Can you work these out from the model? Positions are in its coordinate system, mm. A direction names the side the tool comes from. Coordinates: 2 decimals unless noted, no trailing zeros. Write each loop counter-clockwise with the first axis right and the second up, starting at its lowest first coordinate (ties: lowest second). Pieces come first, ordered by that corner, then holes. Notation, with made-up numbers: M 6,39.5 L 16,39.5 A38 cw 16,78.5 Z; hole C 38.5,-3.75 d11. An arc over 180 degrees is marked long. Use one line per item in the form item = value. Start each with the question number.
```python
from build123d import *

# Parameters (mm, degrees)
SKETCH1_R                = 27.852115
SKETCH1_R_2              = 4
BOSS_EXTRUDE1_DEPTH      = 20
BOSS_EXTRUDE2_DEPTH      = 15
BOSS_EXTRUDE2_DEPTH_BACK = 15
SKETCH2_R                = 2.5
SKETCH4_R                = 1.7
CUT_EXTRUDE1_DEPTH       = 8


with BuildPart() as part:
    # Sketch1 → Boss-Extrude1 (new body)
    with BuildSketch(Plane.XY):
        Circle(SKETCH1_R)
        Circle(SKETCH1_R_2, mode=Mode.SUBTRACT)
    extrude(amount=BOSS_EXTRUDE1_DEPTH)

    # Sketch2 → Boss-Extrude2 (add, two sides: drawn at the far end of the back side and taken through both)
    with BuildSketch(Plane.XY.offset(10).offset(-BOSS_EXTRUDE2_DEPTH_BACK)):
        with Locations((-15, 15)):
            Circle(SKETCH2_R)
        with Locations((15, 15)):
            Circle(SKETCH2_R)
        with Locations((15, -15)):
            Circle(SKETCH2_R)
        with Locations((-15, -15)):
            Circle(SKETCH2_R)
    extrude(amount=BOSS_EXTRUDE2_DEPTH + BOSS_EXTRUDE2_DEPTH_BACK)

    # Sketch4 → Cut-Extrude1 (cut, symmetric)
    with BuildSketch(Plane.XY.offset(10)):
        with Locations((27.852115, 0)):
            Circle(SKETCH4_R)
        with Locations((27.42897879, -4.836469014)):
            Circle(SKETCH4_R)
        with Locations((26.172426939, -9.525984364)):
            Circle(SKETCH4_R)
        with Locations((24.120639139, -13.9260575)):
            Circle(SKETCH4_R)
        with Locations((21.335957925, -17.902994426)):
            Circle(SKETCH4_R)
        with Locations((17.902994426, -21.335957925)):
            Circle(SKETCH4_R)
        with Locations((13.9260575, -24.120639139)):
            Circle(SKETCH4_R)
        with Locations((9.525984364, -26.172426939)):
            Circle(SKETCH4_R)
        with Locations((4.836469014, -27.42897879)):
            Circle(SKETCH4_R)
        with Locations((0, -27.852115)):
            Circle(SKETCH4_R)
        with Locations((-4.836469014, -27.42897879)):
            Circle(SKETCH4_R)
        with Locations((-9.525984364, -26.172426939)):
            Circle(SKETCH4_R)
        with Locations((-13.9260575, -24.120639139)):
            Circle(SKETCH4_R)
        with Locations((-17.902994426, -21.335957925)):
            Circle(SKETCH4_R)
        with Locations((-21.335957925, -17.902994426)):
            Circle(SKETCH4_R)
        with Locations((-24.120639139, -13.9260575)):
            Circle(SKETCH4_R)
        with Locations((-26.172426939, -9.525984364)):
            Circle(SKETCH4_R)
        with Locations((-27.42897879, -4.836469014)):
            Circle(SKETCH4_R)
        with Locations((-27.852115, 0)):
            Circle(SKETCH4_R)
        with Locations((-27.42897879, 4.836469014)):
            Circle(SKETCH4_R)
        with Locations((-26.172426939, 9.525984364)):
            Circle(SKETCH4_R)
        with Locations((-24.120639139, 13.9260575)):
            Circle(SKETCH4_R)
        with Locations((-21.335957925, 17.902994426)):
            Circle(SKETCH4_R)
        with Locations((-17.902994426, 21.335957925)):
            Circle(SKETCH4_R)
        with Locations((-13.9260575, 24.120639139)):
            Circle(SKETCH4_R)
        with Locations((-9.525984364, 26.172426939)):
            Circle(SKETCH4_R)
        with Locations((-4.836469014, 27.42897879)):
            Circle(SKETCH4_R)
        with Locations((0, 27.852115)):
            Circle(SKETCH4_R)
        with Locations((4.836469014, 27.42897879)):
            Circle(SKETCH4_R)
        with Locations((9.525984364, 26.172426939)):
            Circle(SKETCH4_R)
        with Locations((13.9260575, 24.120639139)):
            Circle(SKETCH4_R)
        with Locations((17.902994426, 21.335957925)):
            Circle(SKETCH4_R)
        with Locations((21.335957925, 17.902994426)):
            Circle(SKETCH4_R)
        with Locations((24.120639139, 13.9260575)):
            Circle(SKETCH4_R)
        with Locations((26.172426939, 9.525984364)):
            Circle(SKETCH4_R)
        with Locations((27.42897879, 4.836469014)):
            Circle(SKETCH4_R)
    extrude(amount=CUT_EXTRUDE1_DEPTH, both=True, mode=Mode.SUBTRACT)


solid = part.part
```
1) Please list where these lines run through material, in increasing order: line 1 (X direction, y = -20, z = 16.5); line 2 (Y direction, x = 0, z = 10.75); line 3 (Z direction, x = -2, y = -5).
2) Suppose I cut it at A-A on x = 0. Please give me the cut outline in (y, z), and give its area (3 significant figures).
3) If we mould it in two halves opening along X, with no side actions, what happens to faces 3 (the face through (9, 25, 2)), 4 (the face through (-15, -15, -5)), 5 (the face through (-8.979, 24.563, 9.888))? For each: +X half, -X half, draft (parallel to the pull), parting line (faces both ways), or undercut.
4) Suppose I cut it at B-B on z = -1.25. Please give me the cut outline in (x, y), and give its area (3 significant figures).
5) Which directions (+Z, -Z, +X, -X, +Y, -Y) give clear straight access to the entire face, cutting with the end or side of a thin tool? Please do faces 1 (the face through (-15, -15, 25)), 2 (the face through (22.67, -13.04, 9.89)).
6) Will these pins go through, and if not, where does the flat tip stop? pin 1 Ø0.8 at (x, y) = (-13.5, -24) entering from +Z; pin 2 Ø6 at (x, z) = (-5.5, 17) entering from +Y; pin 3 Ø3 at (x, y) = (20.5, -17.5) entering from -Z.
Computed values:
q1.line_1 = -19.38 to -18.95, -16.85 to 16.85, 18.95 to 19.38
q1.line_2 = -26.15 to -4, 4 to 26.15
q1.line_3 = 0 to 20
q2.outline = M -27.85,0 L -4,0 L -4,20 L -27.85,20 L -27.85,18 L -26.15,18 L -26.15,2 L -27.85,2 Z; M 4,0 L 27.85,0 L 27.85,2 L 26.15,2 L 26.15,18 L 27.85,18 L 27.85,20 L 4,20 Z
q2.area = 900 mm²
q3.face_3 = undercut
q3.face_4 = draft
q3.face_5 = undercut
q4.outline = C -15,-15 d5; C -15,15 d5; C 15,-15 d5; C 15,15 d5
q4.area = 78.5 mm²
q5.face_1 = +Z, +X, -X, +Y, -Y
q5.face_2 = none
q6.pin_1 = 20
q6.pin_2 = 27.74
q6.pin_3 = 0
